Design review of the part built by this model. Coordinates are the model's own, in mm. Face numbers are marked on the shaded views. A direction names the side the tool comes from. Coordinates: 2 decimals unless noted, no trailing zeros. Loops run counter-clockwise (first coordinate to the right, second up) from the corner with the lowest first, then second, coordinate; pieces in that order, holes last. Notation, with made-up numbers: (-28.75, -38.75) - (-1.75, -38.75) arc R38 cw to (-1.75, 0.25) - close; hole circle Ø11 at (13, -20.75). An arc over 180 degrees is marked (long way). Use one line per item in the form item = value. Start each with the question number.
(1) Add section D-D (x = -26). State the section outline as (y, z) points, plus the area to 3 significant figures.
(2) Clearance check with flat-ended pins moving along their axes: pin 1 Ø3.5 at (x, z) = (4, 31) entering from -Y; pin 2 Ø7 at (x, y) = (-15, 9.5) entering from -Z; pin 3 Ø4 at (y, z) = (3, 14) entering from -X; pin 4 Ø6 at (y, z) = (4, 19.5) entering from +X. State where each tip first meets the part, or that it passes through.
(3) Add section C-C (y = -4.25). State the section outline as (x, z) points, plus the area to 3 significant figures.
(4) Tool access review of the marked faces 1, 2, 3, 4 and 5: name each direction out of +Z, -Z, +X, -X, +Y, -Y from which nothing blocks a thin tool from reaching the whole face with its end or side.
(5) Add section A-A (x = -11). State the section outline as (y, z) points.
(6) For L1, parallel to X at y = -0.25, z = 3; L2, parallel to Z at x = 30.5, y = -2; L3, parallel to Y at x = -37.5, z = 28, list the stretches that pass through material, from the lowest coordinate up.
(7) Add section B-B (z = 0). State the section outline as (x, y) points, plus the area to 3 significant figures.
```python
from build123d import *

# Parameters (mm, degrees)
SKETCH_1_W            = 83
SKETCH_1_H            = 48
EXTRUDE_1_DEPTH       = 24
SKETCH_21_W           = 83
SKETCH_21_H           = 1
EXTRUDE_2_DEPTH       = 35.5
CUT_EXTRUDE_20_DEPTH  = 25
MIRROR_2_COPY_1_DEPTH = 25
SKETCH_27_R           = 4
EXTRUDE_4_DEPTH       = 10
SKETCH_28_R           = 0.835314329
SKETCH_28_R_2         = 0.866649433
EXTRUDE_5_DEPTH       = 10


with BuildPart() as part:
    # Sketch 1 → Extrude 1 (new body)
    with BuildSketch(Plane(origin=(0, 18, 0), x_dir=(1, 0, 0), z_dir=(0, 1, 0))):
        Rectangle(SKETCH_1_W, SKETCH_1_H)
    extrude(amount=-EXTRUDE_1_DEPTH)

    # Sketch 21 → Extrude 2 (add, symmetric)
    with BuildSketch(Plane(origin=(0, 0, 0), x_dir=(-1, 0, 0), z_dir=(0, 0, -1))):
        with Locations((0, 17.5)):
            Rectangle(SKETCH_21_W, SKETCH_21_H)
    extrude(amount=EXTRUDE_2_DEPTH, both=True)

    # Sketch 22 → Cut-Extrude 20 (cut, through all)
    with BuildSketch(Plane(origin=(0, 18, 0), x_dir=(-1, 0, 0), z_dir=(0, 1, 0))):
        with BuildLine():
            ThreePointArc((-24, -29.5), (-26, -27.5), (-28, -29.5))
            Line((-28, -29.5), (-24, -29.5))
        make_face()
        with BuildLine():
            Line((-24, -29.5), (-28, -29.5))
            ThreePointArc((-28, -29.5), (-26, -31.5), (-24, -29.5))
        make_face()
        with BuildLine():
            Line((-28, -29.5), (-28, -35.5))
            Line((-28, -35.5), (-24, -35.5))
            Line((-24, -35.5), (-24, -29.5))
            ThreePointArc((-24, -29.5), (-26, -31.5), (-28, -29.5))
        make_face()
    cut_extrude_20 = extrude(amount=-CUT_EXTRUDE_20_DEPTH, mode=Mode.SUBTRACT)

    # Mirror 1: Cut-Extrude 20 across plane
    add(cut_extrude_20.mirror(Plane(origin=(0, 0, 0), x_dir=(0, 0, 1), z_dir=(1, 0, 0))), mode=Mode.SUBTRACT)

    # Mirror 2: Cut-Extrude 20 across plane
    add(cut_extrude_20.mirror(Plane.XY), mode=Mode.SUBTRACT)

    # Mirror 2 copy 1 sketch → Mirror 2 copy 1 (cut, through all)
    with BuildSketch(Plane(origin=(0, 18, 0), x_dir=(1, 0, 0), z_dir=(0, 1, 0))):
        with BuildLine():
            ThreePointArc((-24, -29.5), (-26, -27.5), (-28, -29.5))
            Line((-28, -29.5), (-24, -29.5))
        make_face()
        with BuildLine():
            Line((-24, -29.5), (-28, -29.5))
            ThreePointArc((-28, -29.5), (-26, -31.5), (-24, -29.5))
        make_face()
        with BuildLine():
            Line((-28, -29.5), (-28, -35.5))
            Line((-28, -35.5), (-24, -35.5))
            Line((-24, -35.5), (-24, -29.5))
            ThreePointArc((-24, -29.5), (-26, -31.5), (-28, -29.5))
        make_face()
    extrude(amount=-MIRROR_2_COPY_1_DEPTH, mode=Mode.SUBTRACT)

    # Sketch 27 → Extrude 4 (add)
    with BuildSketch(Plane.ZY.offset(41.5)):
        with Locations((0, 6)):
            Circle(SKETCH_27_R)
    extrude_4 = extrude(amount=EXTRUDE_4_DEPTH)

    # Mirror 3: Extrude 4 across plane
    add(extrude_4.mirror(Plane(origin=(0, 0, 0), x_dir=(0, 0, 1), z_dir=(1, 0, 0))))

    # Sketch 28 → Extrude 5 (add)
    with BuildSketch(Plane(origin=(41.5, 0, 0), x_dir=(0, 0, -1), z_dir=(1, 0, 0))):
        with Locations((-19.628552742, 6.499481813)):
            Circle(SKETCH_28_R)
        with Locations((-16.419283225, 6.499481813)):
            Circle(SKETCH_28_R_2)
    extrude(amount=EXTRUDE_5_DEPTH)


solid = part.part
```
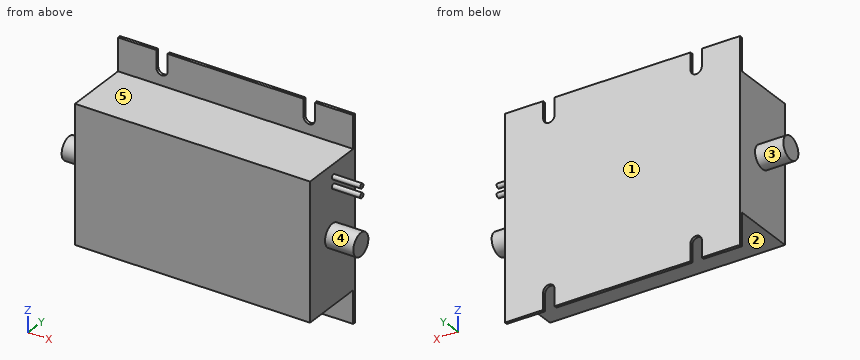
Computed values:
q1.outline = (-6, -24) - (17, -24) - (17, -27.5) - (18, -27.5) - (18, 27.5) - (17, 27.5) - (17, 24) - (-6, 24) - close
q1.area = 1,160 mm^2
q2.pin_1 = 17
q2.pin_2 = -24
q2.pin_3 = -41.5
q2.pin_4 = 51.5
q3.outline = (-41.5, -24) - (41.5, -24) - (41.5, 24) - (-41.5, 24) - close
q3.area = 3,980 mm^2
q4.face_1 = +Z, -Z, +X, -X, +Y
q4.face_2 = -Z, +X, -X, -Y
q4.face_3 = -X
q4.face_4 = +X
q4.face_5 = +Z, +X, -X, -Y
q5.outline = (-6, -24) - (17, -24) - (17, -35.5) - (18, -35.5) - (18, 35.5) - (17, 35.5) - (17, 24) - (-6, 24) - close
q6.L1 = -41.5 to 41.5
q6.L2 = -24 to 24
q6.L3 = 17 to 18
q7.outline = (-51.5, 2) - (-41.5, 2) - (-41.5, -6) - (41.5, -6) - (41.5, 2) - (51.5, 2) - (51.5, 10) - (41.5, 10) - (41.5, 18) - (-41.5, 18) - (-41.5, 10) - (-51.5, 10) - close
q7.area = 2,150 mm^2
